For this review, use the dimensioned drawing (mm, ordinates from the lowest corner) and the shaded views. Give positions to 0.01 mm unless a question says otherwise; leave off trailing zeros. Order: outer loops, then holes, each group sorted by start corner. A loop starts at its lowest first (then second) coordinate and runs counter-clockwise, first axis right, second up.
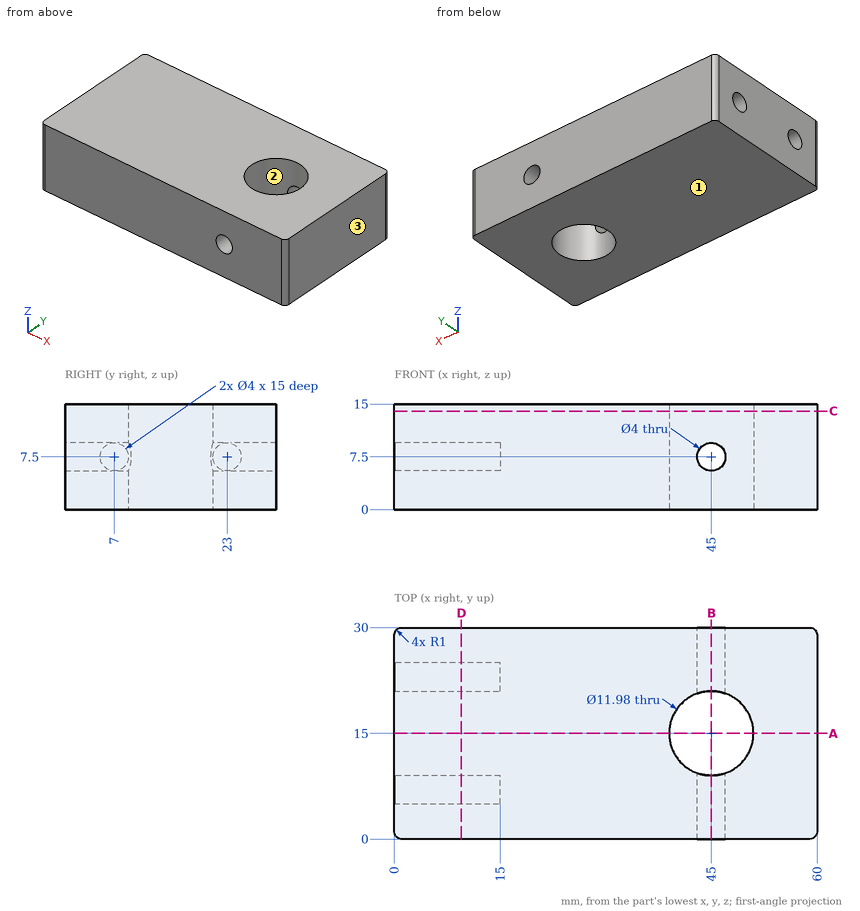
1. Take a section at C-C (z = 14). State the section outline as (x, y) points, then the cut area to 3 significant figures.
Recorded:
outline: (0, 1) arc R1 ccw to (1, 0) - (59, 0) arc R1 ccw to (60, 1) - (60, 29) arc R1 ccw to (59, 30) - (1, 30) arc R1 ccw to (0, 29) - close; hole circle Ø11.98 at (45, 15)
area: 1,690 mm2
2. For line 1 along Y through (x, z) = (43, 2.25); line 2 along Z through (x, y) = (10.25, 7); line 3 along X through (y, z) = (3.25, 7.5), list the stretches that pass through material, from the lowest coordinate up.
Recorded:
line 1: y = 0 to 9.35, 20.65 to 30
line 2: z = 0 to 5.5, 9.5 to 15
line 3: x = 0 to 43, 47 to 60
3. For pin 1 (1.2 mm diameter, centred on y = 6.5, z = 7, fed in from -X), flat-tipped, find the tip position at first contact; note if it passes through.
Recorded:
pin 1: stops at x = 15
4. Take a section at A-A (y = 15). State the section outline as (x, z) points.
Recorded:
outline: (0, 0) - (39.01, 0) - (39.01, 15) - (0, 15) - close; (50.99, 0) - (60, 0) - (60, 15) - (50.99, 15) - close
5. Draft analysis for pull direction X (two halves, no side actions). For the marked faces 1, 2 and 3, state which applies: pulls with the +X half, pulls with the -X half, needs draft (parallel to the pull), parting line crosses it, or undercut.
Recorded:
face 1: needs draft
face 2: undercut
face 3: pulls with the +X half
6. Take a section at D-D (x = 9.5). State the section outline as (y, z) points.
Recorded:
outline: (0, 0) - (30, 0) - (30, 15) - (0, 15) - close; hole circle Ø4 at (7, 7.5); hole circle Ø4 at (23, 7.5)
7. Take a section at B-B (x = 45). State the section outline as (y, z) points.
Recorded:
outline: (0, 0) - (9.01, 0) - (9.01, 5.5) - (0, 5.5) - close; (0, 9.5) - (9.01, 9.5) - (9.01, 15) - (0, 15) - close; (20.99, 0) - (30, 0) - (30, 5.5) - (20.99, 5.5) - close; (20.99, 9.5) - (30, 9.5) - (30, 15) - (20.99, 15) - close
